Can you work these out from the model? Positions are in its coordinate system, mm. A direction names the side the tool comes from. Give positions to 0.01 mm unless a question says otherwise; leave off trailing zeros. Loops run counter-clockwise (first coordinate to the right, second up) from the corner with the lowest first, then second, coordinate; pieces in that order, holes last. Notation, with made-up numbers: (11, 29.5) - (20, 29.5) arc R15 cw to (20, 50.5) - close; hole circle Ø4 at (72, 31). An arc over 180 degrees is marked (long way). Answer as a JSON object with one key per item and string values. Group by question number.
Item 1: Suppose I cut it at B-B on z = 18. Write out the boundary of the cut face in (x, y).
Item 2: Suppose I cut it at C-C on x = 16.25. Write out the boundary of the cut face in (y, z).
Item 3: Thinking about a two-plate mould opening in Z: for faces 1 (the flat face through (4, -6, 21.46)), 2 (the flat face through (16, -8, 18)), 3 (the flat face through (4, -6, 14.51)), which applies, pulls with the +Z half, pulls with the -Z half, needs draft (parallel to the pull), parting line crosses it, or undercut?
Item 4: Suppose I cut it at D-D on y = -14.25. Write out the boundary of the cut face in (x, z), and give its area (3 significant figures).
Item 5: Will these pins go through, and if not, where does the flat tip stop? pin 1 (3.5 mm diameter, centred on y = -7, z = 18, fed in from -X); pin 2 (5 mm diameter, centred on x = 15, y = -12, fed in from +Z); pin 3 (1.2 mm diameter, centred on x = 16.5, z = 19.5, fed in from -Y).
Item 6: Please list where these lines run through material, in increasing order: L1, parallel to Y at x = 5, z = 6; L2, parallel to Z at x = 4, y = -15.
Item 7: Suppose I cut it at A-A on y = -5.75. Write out the boundary of the cut face in (x, z).
Item 8: Which directions (+Z, -Z, +X, -X, +Y, -Y) give clear straight access to the entire face, cutting with the end or side of a thin tool? Please do faces 4 (the flat face through (17.65, -6, 18)), 5 (the flat face through (4, -8, 18)), 6 (the flat face through (2.35, -6, 18)).
from build123d import *

# Parameters (mm, degrees)
F0_W     = 20
F0_H     = 25
F1_DEPTH = 5
F2_W     = 20
F2_H     = 3
F3_DEPTH = 15
F4_W     = 2.4
F4_H     = 6.95
F5_DEPTH = 3


with BuildPart() as f1:
    # F0 (on Front) → F1 (new body)
    with BuildSketch(Plane.XZ):
        with Locations((10, 12.5)):
            Rectangle(F0_W, F0_H)
    extrude(amount=F1_DEPTH)

    # F2 (on face) → F3 (join)
    with BuildSketch(Plane.XZ.offset(5)):
        with Locations((10, 1.5)):
            Rectangle(F2_W, F2_H)
    extrude(amount=F3_DEPTH)

    # F4 (on face) → F5 (join)
    with BuildSketch(Plane.XZ.offset(5)):
        with Locations((3.55, 17.985)):
            Rectangle(F4_W, F4_H)
        with Locations((16.45, 17.985)):
            Rectangle(F4_W, F4_H)
    extrude(amount=F5_DEPTH)


solid = f1.part
Worked out:
{
 "1": {"outline": "(0, -5) - (2.35, -5) - (2.35, -8) - (4.75, -8) - (4.75, -5) - (15.25, -5) - (15.25, -8) - (17.65, -8) - (17.65, -5) - (20, -5) - (20, 0) - (0, 0) - close"},
 "2": {"outline": "(-20, 0) - (0, 0) - (0, 25) - (-5, 25) - (-5, 21.46) - (-8, 21.46) - (-8, 14.51) - (-5, 14.51) - (-5, 3) - (-20, 3) - close"},
 "3": {"face 1": "pulls with the +Z half", "face 2": "needs draft", "face 3": "undercut"},
 "4": {"outline": "(0, 0) - (20, 0) - (20, 3) - (0, 3) - close", "area": "60.0 mm2"},
 "5": {"pin 1": "stops at x = 2.35", "pin 2": "stops at z = 3", "pin 3": "stops at y = -8"},
 "6": {"L1": "y = -5 to 0", "L2": "z = 0 to 3"},
 "7": {"outline": "(0, 0) - (20, 0) - (20, 3) - (0, 3) - close; (2.35, 14.51) - (4.75, 14.51) - (4.75, 21.46) - (2.35, 21.46) - close; (15.25, 14.51) - (17.65, 14.51) - (17.65, 21.46) - (15.25, 21.46) - close"},
 "8": {"face 4": "+Z, +X, -Y", "face 5": "+Z, +X, -X, -Y", "face 6": "+Z, -X, -Y"}
}
